```python
from build123d import *

# Parameters (mm, degrees)
SKETCH1_R           = 2.032
BOSS_EXTRUDE1_DEPTH = 3.175
SKETCH2_R           = 5.715
CUT_EXTRUDE1_DEPTH  = 3.175
BOSS_EXTRUDE2_START = 25.4
SKETCH3_R           = 14.605
SKETCH3_R_2         = 5.715
BOSS_EXTRUDE2_DEPTH = 25.4
SKETCH6_R           = 8.845512053
CUT_EXTRUDE3_DEPTH  = 22.225
CUT_EXTRUDE5_DEPTH  = 3.175


with BuildPart() as part:
    # Sketch1 → Boss-Extrude1 (new body)
    with BuildSketch(Plane.XY):
        with BuildLine():
            Line((0.092337824, 22.85981351), (0.092337824, 40.89418649))
            ThreePointArc((0.092337824, 40.89418649), (16.63628773, 48.075558414), (22.825148771, 65.015817568))
            Line((22.825148771, 65.015817568), (40.859521751, 65.015817568))
            ThreePointArc((40.859521751, 65.015817568), (47.048382792, 48.075558414), (63.592332697, 40.89418649))
            Line((63.592332697, 40.89418649), (63.592332697, 22.85981351))
            ThreePointArc((63.592332697, 22.85981351), (47.048382792, 15.678441586), (40.859521751, -1.261817568))
            Line((40.859521751, -1.261817568), (22.825148771, -1.261817568))
            ThreePointArc((22.825148771, -1.261817568), (16.63628773, 15.678441586), (0.092337824, 22.85981351))
        make_face()
        with Locations((6.442335261, 31.877)):
            Circle(SKETCH1_R, mode=Mode.SUBTRACT)
        with Locations((31.842335261, 57.277)):
            Circle(SKETCH1_R, mode=Mode.SUBTRACT)
        with Locations((57.242335261, 31.877)):
            Circle(SKETCH1_R, mode=Mode.SUBTRACT)
        with Locations((31.842337824, 6.477)):
            Circle(SKETCH1_R, mode=Mode.SUBTRACT)
    extrude(amount=BOSS_EXTRUDE1_DEPTH)

    # Sketch2 → Cut-Extrude1 (cut)
    with BuildSketch(Plane.XY.offset(3.175)):
        with Locations((31.415168912, 31.877)):
            Circle(SKETCH2_R)
    extrude(amount=-CUT_EXTRUDE1_DEPTH, mode=Mode.SUBTRACT)

    # Sketch3 → Boss-Extrude2 (add)
    with BuildSketch(Plane.XY.offset(3.175).offset(BOSS_EXTRUDE2_START)):
        with Locations((31.415168912, 31.877)):
            Circle(SKETCH3_R)
        with Locations((31.415168912, 31.877)):
            Circle(SKETCH3_R_2, mode=Mode.SUBTRACT)
    extrude(amount=-BOSS_EXTRUDE2_DEPTH)

    # Sketch6 → Cut-Extrude3 (cut)
    with BuildSketch(Plane.XY.offset(28.575)):
        with Locations((31.415168912, 31.877)):
            Circle(SKETCH6_R)
    extrude(amount=-CUT_EXTRUDE3_DEPTH, mode=Mode.SUBTRACT)

    # Sketch7 → Cut-Extrude5 (cut)
    with BuildSketch(Plane(origin=(0, 0, 0), x_dir=(-1, 0, 0), z_dir=(0, 0, -1))):
        Polygon((-23.056493238, 31.877), (-27.235831075, 39.115825476), (-35.594506749, 39.115825476), (-39.773844587, 31.877), (-35.594506749, 24.638174524), (-27.235831075, 24.638174524), align=None)
    extrude(amount=-CUT_EXTRUDE5_DEPTH, mode=Mode.SUBTRACT)


solid = part.part
```
CAD build for the part. Positions are in the model's coordinates, mm. A direction names the side the tool comes from. Round coordinates to 2 decimals unless told otherwise and drop trailing zeros. Order: outer loops, then holes, each group sorted by start corner. A loop starts at its lowest first (then second) coordinate and runs counter-clockwise, first axis right, second up.
Q1. Slice it at C-C (x = 31). Write the cut outline in (y, z) (3 decimals), and give its area (3 significant figures).
Q2. Drop flat-ended pins along their axis: pin 1 (7 mm diameter, centred on x = 31.42, y = 31.88, fed in from -Z); pin 2 (10 mm diameter, centred on x = 43.5, z = 13.5, fed in from -Y); pin 3 (7 mm diameter, centred on x = 31.5, y = 34.5, fed in from -Z) (3 decimals); pin 4 (4 mm diameter, centred on y = 27.5, z = 23.5, fed in from -X). Give the stop position or say it passes through.
Q3. Wall check: L1, parallel to Z at x = 42.5, y = 19 (3 decimals); L2, parallel to Y at x = 28, z = 1.5; L3, parallel to X at y = 32.5, z = 24.75. Give the ranges that are in metal, low to high.
Q4. Slice it at D-D (y = 19). Write the cut outline in (x, z) (3 decimals).
Q5. Slice it at B-B (z = 20.5). Write the cut outline in (x, y) (3 decimals).
Q6. Slice it at A-A (x = 57.5). Write the cut outline in (y, z) (3 decimals).
Q7. Which spindle directions (+Z, -Z, +X, -X, +Y, -Y) get a long thin tool onto all of the face, cutting with end or side? Do faces 1 (the flat face through (31, 26, 6.35)), 2 (the flat face through (25.12, 35.45, 1.57)), 3 (the flat face through (32, 40, 0)). Say none if no direction does.
Q8. Two-plate mould, pull along Y, no slides. Class faces 4 (the cylindrical face through (34.488, 36.696, 4.785)), 5 (the flat face through (32, -1.262, 2)), 6 (the flat face through (46.4, 32.3, 3.175)): pulls with the +Y half, pulls with the -Y half, needs draft (parallel to the pull), parting line crosses it, or undercut.
Results below:
1. outline: (-1.262, 0) - (4.628, 0) - (4.628, 3.175) - (-1.262, 3.175) - close; (8.326, 0) - (24.638, 0) - (24.638, 3.175) - (26.177, 3.175) - (26.177, 6.35) - (23.041, 6.35) - (23.041, 28.575) - (17.278, 28.575) - (17.278, 3.175) - (8.326, 3.175) - close; (37.577, 3.175) - (39.116, 3.175) - (39.116, 0) - (55.428, 0) - (55.428, 3.175) - (46.476, 3.175) - (46.476, 28.575) - (40.713, 28.575) - (40.713, 6.35) - (37.577, 6.35) - close; (59.126, 0) - (65.016, 0) - (65.016, 3.175) - (59.126, 3.175) - close
1. area: 454 mm2
2. pin 1: passes through
2. pin 2: stops at y = 19.11
2. pin 3: stops at z = 3.175
2. pin 4: stops at x = 17
3. L1: z = 0 to 3.175
3. L2: y = -1.26 to 24.64, 39.12 to 65.02
3. L3: x = 16.82 to 22.59, 40.24 to 46.01
4. outline: (12.711, 0) - (50.973, 0) - (50.973, 3.175) - (38.306, 3.175) - (38.306, 28.575) - (24.524, 28.575) - (24.524, 3.175) - (12.711, 3.175) - close
5. outline: circle Ø29.21 at (31.415, 31.877); hole circle Ø17.691 at (31.415, 31.877)
6. outline: (22.007, 0) - (29.861, 0) - (29.861, 3.175) - (22.007, 3.175) - close; (33.893, 0) - (41.747, 0) - (41.747, 3.175) - (33.893, 3.175) - close
7. face 1: +Z
7. face 2: -Z
7. face 3: -Z, +X, -X, +Y, -Y
8. face 4: undercut
8. face 5: pulls with the -Y half
8. face 6: needs draft
